Autodesk Inventor part; units mm, degrees
ref_plane "YZ Plane" through (0, 0, 0) normal (1, 0, 0) x (0, 1, 0)
ref_plane "XZ Plane" through (0, 0, 0) normal (0, 1, 0) x (-1, 0, 0)
ref_plane "XY Plane" through (0, 0, 0) normal (0, 0, 1) x (1, 0, 0)
sketch "Sketch1" plane through (0, 0, 0) normal (0, 1, 0) x (-1, 0, 0)
  line L0 (0, 0) -> (19.177, 0)
  line L1 (19.177, 0) -> (19.177, -14.478)
  line L2 (19.177, -14.478) -> (0, -14.478)
  line L3 (0, -14.478) -> (0, 0)
  dimension "d0" = 19.177
  dimension "d1" = 14.478
extrude "Extrusion1" add sketch "Sketch1" along normal blind 8.89
sketch "Sketch2" plane through (0, 0, 0) normal (1, 0, 0) x (0, 0, -1)
  circle A0 centre (7.239, 4.445) radius 9.4742
  line L0 (0, 8.89) -> (14.478, 8.89)
  line L1 (0, 0) -> (0, 8.89)
  line L2 (14.478, 0) -> (0, 0)
  line L3 (0, 0) -> (0, 8.89)
  point P0 (7.239, 0)
  point P1 (0, 4.445)
  dimension "d4" = 18.9484
  dimension "d9" = 0
  dimension "d10" = 0
extrude "Extrusion2" add sketch "Sketch2" along normal blind 40.005
fillet "Fillet1" radius 3.175 2 edges at (-19.177, 4.445, 0) (-19.177, 4.445, -14.478)
properties part number "Part6 x 2"
The listing builds one solid part. Answer for the finished solid, in the listing's coordinates (mm). A direction names the side the tool comes from. Round coordinates to 2 decimals unless told otherwise and drop trailing zeros. Write each loop counter-clockwise with the first axis right and the second up, starting at its lowest first coordinate (ties: lowest second). Pieces come first, ordered by that corner, then holes. Notation, with made-up numbers: (7, 69.5) -> (32, 69.5) arc R15 ccw to (32, 92.5) -> close; hole circle Ø1 at (38, 76). An arc over 180 degrees is marked (long way). Use CSV: the item, a comma, the result in double quotes. Start each with the question number.
(1) Which of the six approach directions +Z, -Z, +X, -X, +Y, -Y give full straight-line access (tool end or side, diameter ignored) to faces 1 (the face through (-8, 4, 0)), 2 (the face through (-9, 8.89, -7)), 3 (the face through (-8, 4, -14.478)), 4 (the face through (40.005, 5, -7)), 5 (the face through (-9, 0, -7))?
(2) Section D-D on y = 3.5 is taken. Give the vertices of the cut face in (x, z) (3 decimals).
(3) Section C-C on x = -6 is taken. Give the vertices of the cut face in (y, z), then the cut area to 3 significant figures.
(4) Section A-A on z = -13.75 is taken. Give the vertices of the cut face in (x, y) (3 decimals).
(5) Consider L1, parallel to X at y = -0.5, z = -5 (3 decimals); L2, parallel to Y at x = -15.5, z = -7; L3, parallel to Y at x = 37.5, z = -9.75. Determine where each line is inside the solid, lowest interval first. Write a range as from..to.
(6) Each of these flat-tipped pins is pushed along its axis until it touches: pin 1 (10 mm diameter, centred on x = -6, y = 4.5, fed in from +Z); pin 2 (5.5 mm diameter, centred on y = 3.5, z = -11.5, fed in from -X); pin 3 (4 mm diameter, centred on x = 18, z = -9.5, fed in from -Y); pin 4 (1.5 mm diameter, centred on x = 1.5, z = -9, fed in from +Y). Where does it stop, or does it pass through?
(7) Section B-B on y = 8.25 is taken. Give the vertices of the cut face in (x, z) (3 decimals).
A:
1,face 1,"+Z, -X, +Y, -Y"
1,face 2,"+Z, -Z, -X, +Y"
1,face 3,"-Z, -X, +Y, -Y"
1,face 4,"+Z, -Z, +X, +Y, -Y"
1,face 5,"+Z, -Z, -X, -Y"
2,outline,"(-19.177, -11.303) arc R3.175 ccw to (-16.002, -14.478) -> (0, -14.478) -> (0, -16.666) -> (40.005, -16.666) -> (40.005, 2.188) -> (0, 2.188) -> (0, 0) -> (-16.002, 0) arc R3.175 ccw to (-19.177, -3.175) -> close"
3,outline,"(0, -14.48) -> (8.89, -14.48) -> (8.89, 0) -> (0, 0) -> close"
3,area,"129 mm²"
4,outline,"(-18.025, 0) -> (0, 0) -> (0, -2.437) -> (40.005, -2.437) -> (40.005, 11.327) -> (0, 11.327) -> (0, 8.89) -> (-18.025, 8.89) -> close"
5,L1,"x = 0..40.005"
5,L2,"y = 0..8.89"
5,L3,"y = -4.69..13.58"
6,pin 1,"stops at z = 0"
6,pin 2,"stops at x = -19.18"
6,pin 3,"stops at y = -5.03"
6,pin 4,"stops at y = 13.87"
7,outline,"(-19.177, -11.303) arc R3.175 ccw to (-16.002, -14.478) -> (0, -14.478) -> (0, -15.916) -> (40.005, -15.916) -> (40.005, 1.438) -> (0, 1.438) -> (0, 0) -> (-16.002, 0) arc R3.175 ccw to (-19.177, -3.175) -> close"
